CAD build for the part. Positions are in the model's coordinates, mm. A direction names the side the tool comes from. Coordinates: 2 decimals unless noted, no trailing zeros. Write each loop counter-clockwise with the first axis right and the second up, starting at its lowest first coordinate (ties: lowest second). Pieces come first, ordered by that corner, then holes.
```python
from build123d import *

# Parameters (mm, degrees)
ESQUISSE1_R        = 5.5
BOSS_EXTRU_1_DEPTH = 12
ESQUISSE2_W        = 12
ESQUISSE2_H        = 3
BOSS_EXTRU_2_DEPTH = 7
BOSS_EXTRU_3_DEPTH = 12
CHANFREIN1_SIZE    = 2
CONG_1_R           = 1


with BuildPart() as part:
    # Esquisse1 → Boss.-Extru.1 (new body)
    with BuildSketch(Plane.XY):
        with Locations((25.477220372, 0.406206053)):
            Circle(ESQUISSE1_R)
    extrude(amount=BOSS_EXTRU_1_DEPTH)

    # Esquisse2 → Boss.-Extru.2 (add)
    with BuildSketch(Plane.XY.offset(2.5)):
        with Locations((19.654430588, 4.343698911)):
            Rectangle(ESQUISSE2_W, ESQUISSE2_H)
    extrude(amount=BOSS_EXTRU_2_DEPTH)

    # Esquisse3 → Boss.-Extru.3 (add)
    with BuildSketch(Plane.XY):
        Polygon((-49.298156478, 2.843698911), (13.654430588, 2.843698911), (13.654430588, 5.843698911), (-56.345569412, 5.843698911), (-56.345569412, 2.843698911), (-51.345569412, 2.843698911), (-51.345569412, -7.156301089), (-46.345569412, -7.156301089), (-46.345569412, -5.156301089), (-49.298156478, -5.156301089), align=None)
    extrude(amount=BOSS_EXTRU_3_DEPTH)

    # Chanfrein1
    chanfrein1_edges = [part.edges().sort_by_distance(p)[0] for p in [
        (-51.345569412, -7.156301089, 6),
    ]]
    chamfer(chanfrein1_edges, length=CHANFREIN1_SIZE)

    # Congé1
    cong_1_edges = [part.edges().sort_by_distance(p)[0] for p in [
        (-56.345569412, 5.843698911, 6),
        (-56.345569412, 2.843698911, 6),
    ]]
    fillet(cong_1_edges, radius=CONG_1_R)


solid = part.part
```
Item 1: Wall check: line 1 along X through (y, z) = (0.5, 1.75); line 2 along Y through (x, z) = (-47.5, 2.5); line 3 along Y through (x, z) = (-18.5, 3.75). Give the ranges that are in metal, low to high.
Item 2: Which spindle directions (+Z, -Z, +X, -X, +Y, -Y) get a long thin tool onto all of the face, cutting with end or side? Do faces 4 (the flat face through (18, 4, 9.5)), 5 (the flat face through (-53, 2.844, 6)), 6 (the flat face through (-48, -5.156, 6)), 7 (the flat face through (-49.298, -1, 6)). Say none if no direction does.
Item 3: Two-plate mould, pull along X, no slides. Class faces 1 (the flat face through (-46.346, -6, 6)), 2 (the flat face through (-48, -7.156, 6)), 3 (the flat face through (18, 4, 2.5)): +X half, -X half, draft (parallel to the pull), parting line (faces both ways), or undercut.
Item 4: Flat gauge pins, fed straight in: pin 1 Ø0.8 at (y, z) = (5, 1) entering from +X; pin 2 Ø4 at (y, z) = (-2, 8) entering from +X; pin 3 Ø6 at (x, z) = (-4, 3) entering from -Y. Where does each tip first touch, or does it go through?
Item 5: Saw through at B-B, the plane y = 1.5. Write the cut outline in (x, z), and give its area (3 significant figures).
Item 6: Saw through at A-A, the plane z = 8.75. Write the cut outline in (x, y), and give its area (3 significant figures).
Item 7: Saw through at C-C, the plane x = -11. Write the cut outline in (y, z), and give its area (3 significant figures).
Item 8: Saw through at D-D, the plane z = 1. Write the cut outline in (x, y), and give its area (3 significant figures).
Working result:
1. line 1: x = -51.35 to -49.3, 19.98 to 30.98
1. line 2: y = -7.16 to -5.16, 2.84 to 5.84
1. line 3: y = 2.84 to 5.84
2. face 4: +Z, +Y
2. face 5: +Z, -Z, -X, -Y
2. face 6: +Z, -Z, +X
2. face 7: +Z, -Z
3. face 1: +X half
3. face 2: draft
3. face 3: undercut
4. pin 1: stops at x = 29.04
4. pin 2: stops at x = 30.96
4. pin 3: stops at y = 2.84
5. outline: (-51.35, 0) - (-49.3, 0) - (-49.3, 12) - (-51.35, 12) - close; (20.09, 0) - (30.87, 0) - (30.87, 12) - (20.09, 12) - close
5. area: 154 mm2
6. outline: (-56.35, 3.84) arc R1 ccw to (-55.35, 2.84) - (-51.35, 2.84) - (-51.35, -5.16) - (-49.35, -7.16) - (-46.35, -7.16) - (-46.35, -5.16) - (-49.3, -5.16) - (-49.3, 2.84) - (20.55, 2.84) arc R5.5 ccw (long way) to (24.65, 5.84) - (-55.35, 5.84) arc R1 ccw to (-56.35, 4.84) - close
6. area: 354 mm2
7. outline: (2.84, 0) - (5.84, 0) - (5.84, 12) - (2.84, 12) - close
7. area: 36.0 mm2
8. outline: (-56.35, 3.84) arc R1 ccw to (-55.35, 2.84) - (-51.35, 2.84) - (-51.35, -5.16) - (-49.35, -7.16) - (-46.35, -7.16) - (-46.35, -5.16) - (-49.3, -5.16) - (-49.3, 2.84) - (13.65, 2.84) - (13.65, 5.84) - (-55.35, 5.84) arc R1 ccw to (-56.35, 4.84) - close; circle Ø11 at (25.48, 0.41)
8. area: 329 mm2
